from build123d import *

# Parameters (mm, degrees)
F0_W     = 230
F0_H     = 100
F1_DEPTH = 10
F2_R     = 35
F3_DEPTH = 41
F4_R     = 10
F5_DEPTH = 300


with BuildPart() as f1:
    # F0 (on Front) → F1 (new body)
    with BuildSketch(Plane.XZ):
        Rectangle(F0_W, F0_H)
    extrude(amount=F1_DEPTH)

    # F2 (on face) → F3 (join)
    with BuildSketch(Plane.XZ.offset(10)):
        with Locations((-75, 0)):
            Circle(F2_R)
        with Locations((75, 0)):
            Circle(F2_R)
    extrude(amount=F3_DEPTH)

    # F4 (on face) → F5 (join)
    with BuildSketch(Plane.XZ.offset(51)):
        with Locations((-75, 0)):
            Circle(F4_R)
        with Locations((75, 0)):
            Circle(F4_R)
    extrude(amount=F5_DEPTH)


solid = f1.part
The model under review builds one solid part; all positions refer to its coordinate system, in mm. A direction names the side the tool comes from. Coordinates: 2 decimals unless noted, no trailing zeros. Loops run counter-clockwise (first coordinate to the right, second up) from the corner with the lowest first, then second, coordinate; pieces in that order, holes last. Notation, with made-up numbers: (-11.5, 52) -> (32.5, 52) arc R24 ccw to (32.5, 82) -> close; hole circle Ø6 at (-3.75, -18.5). An arc over 180 degrees is marked (long way). Use a Markdown table: item, result. Add a question column.
1. To check wall thickness, follow line 1 (Y direction, x = -7.5, z = -38); line 2 (Y direction, x = 87, z = -2.5); line 3 (Z direction, x = -66, y = -275.5). State the ranges of each line that lie inside material, in increasing order.
2. Draft analysis for pull direction X (two halves, no side actions). For faces 1 (the face through (-42.67, -30.21, -13.41)), 2 (the face through (65, -199, 0)), 3 (the face through (-115, -5, -1)), 4 (the face through (75, -351, 0)), state which applies: pulls with the +X half, pulls with the -X half, needs draft (parallel to the pull), parting line crosses it, or undercut.
3. Machinability: for faces 5 (the face through (115, -5, -1)), 6 (the face through (-85, -199, 0)), which of the approach directions +Z, -Z, +X, -X, +Y, -Y give a long, thin tool a straight path to every point of the face, cutting with its end or side? Answer none if there is none.
4. Add section C-C on x = 75. Write out the cut boundary in (y, z), plus the area to 3 significant figures.
5. Add section A-A on y = -189.5. Write out the cut boundary in (x, z), plus the area to 3 significant figures.
6. Clearance check with flat-ended pins moving along their axes: pin 1 Ø2 at (x, y) = (-82, -279.5) entering from +Z; pin 2 Ø1 at (x, y) = (-85.5, -37.5) entering from +Z; pin 3 Ø12 at (x, z) = (-78, 37.5) entering from +Y; pin 4 Ø10 at (x, z) = (73, 34.5) entering from -Y. State where each tip first meets the part, or that it passes through.
7. Add section B-B on z = 0. Write out the cut boundary in (x, y), plus the area to 3 significant figures.
8. Add section D-D on x = -91. Write out the cut boundary in (y, z).
Returned:
| question | item | result |
|---|---|---|
| 1 | line 1 | y = -10 to 0 |
| 1 | line 2 | y = -51 to 0 |
| 1 | line 3 | z = -4.36 to 4.36 |
| 2 | face 1 | undercut |
| 2 | face 2 | undercut |
| 2 | face 3 | pulls with the -X half |
| 2 | face 4 | needs draft |
| 3 | face 5 | +Z, -Z, +X, +Y, -Y |
| 3 | face 6 | -Y |
| 4 | outline | (-351, -10) -> (-51, -10) -> (-51, -35) -> (-10, -35) -> (-10, -50) -> (0, -50) -> (0, 50) -> (-10, 50) -> (-10, 35) -> (-51, 35) -> (-51, 10) -> (-351, 10) -> close |
| 4 | area | 9,870 mm² |
| 5 | outline | circle Ø20 at (-75, 0); circle Ø20 at (75, 0) |
| 5 | area | 628 mm² |
| 6 | pin 1 | stops at z = 8 |
| 6 | pin 2 | stops at z = 33.54 |
| 6 | pin 3 | stops at y = 0 |
| 6 | pin 4 | stops at y = -51 |
| 7 | outline | (-115, -10) -> (-110, -10) -> (-110, -51) -> (-85, -51) -> (-85, -351) -> (-65, -351) -> (-65, -51) -> (-40, -51) -> (-40, -10) -> (40, -10) -> (40, -51) -> (65, -51) -> (65, -351) -> (85, -351) -> (85, -51) -> (110, -51) -> (110, -10) -> (115, -10) -> (115, 0) -> (-115, 0) -> close |
| 7 | area | 20,000 mm² |
| 8 | outline | (-51, -31.13) -> (-10, -31.13) -> (-10, -50) -> (0, -50) -> (0, 50) -> (-10, 50) -> (-10, 31.13) -> (-51, 31.13) -> close |
